Autodesk Inventor part; units mm, degrees
ref_plane "YZ Plane" through (0, 0, 0) normal (1, 0, 0) x (0, 1, 0)
ref_plane "XZ Plane" through (0, 0, 0) normal (0, 1, 0) x (-1, 0, 0)
ref_plane "XY Plane" through (0, 0, 0) normal (0, 0, 1) x (1, 0, 0)
sketch "Sketch1" plane through (0, 0, 0) normal (0, 1, 0) x (-1, 0, 0)
  line L0 (0, 0) -> (0, -90)
  line L1 (0, -90) -> (-5, -90)
  line L2 (-5, -90) -> (-5, -87.5)
  line L3 (-5, -82.5) -> (-5, -7.5)
  line L4 (-5, -7.5) -> (-7.5, -9)
  line L5 (-7.5, -9) -> (-7.5, -1)
  line L6 (-7.5, -1) -> (-5, -2.5)
  line L7 (-5, -2.5) -> (-5, 0)
  line L8 (-5, 0) -> (0, 0)
  line L9 (-5, -7.5) -> (-5, -2.5) construction
  line L10 (-5, -82.5) -> (-5, -87.5) construction
  line L11 (0, -45) -> (-5, -45) construction
  line L12 (-5, -82.5) -> (-7.5, -81)
  line L13 (-7.5, -81) -> (-7.5, -89)
  line L14 (-7.5, -89) -> (-5, -87.5)
  line L15 (0, 0) -> (-10, 0)
  line L16 (-10, 0) -> (-10, -10)
  line L17 (-10, -10) -> (0, -10)
  line L18 (0, -10) -> (0, 0)
  line L19 (0, -90) -> (-10, -90)
  line L20 (-10, -90) -> (-10, -80)
  line L21 (-10, -80) -> (0, -80)
  line L22 (0, -80) -> (0, -90)
  point P0 (-7.5, -5)
  point P1 (-5, -5)
  point P2 (-5, -85)
  point P3 (0, -80)
  point P4 (-5, 0)
  point P5 (0, -10)
  point P6 (-5, -80)
  dimension "d0" = 90
  dimension "d1" = 5
  dimension "d2" = 8
  dimension "d3" = 5
  dimension "d4" = 5
  dimension "d5" = 2.5
  dimension "d6" = 5
  dimension "d9" = 5
  dimension "d10" = 10
  dimension "d11" = 10
  dimension "d12" = 10
  dimension "d13" = 10
extrude "Extrusion1" add sketch "Sketch1" along normal blind 3 contours L0 L17 L3 L4 L5 L6 L7 L8 | L7 L6 L5 L4 L3 L17 L16 L15 | L0 L1 L2 L14 L13 L12 L3 L21 | L3 L12 L13 L14 L2 L19 L20 L21
extrude "Extrusion2" add sketch "Sketch1" along normal blind 80 contours L0 L17 L3 L4 L5 L6 L7 L8 | L0 L21 L3 L17 | L0 L1 L2 L14 L13 L12 L3 L21
sketch "Sketch2" plane through (0, 0, 0) normal (0, 0, 1) x (1, 0, 0)
  line L0 (0, 0) -> (0, 80)
  line L1 (0, 13.75) -> (2.5, 13.75)
  line L2 (2.5, 13.75) -> (2.5, 16.25)
  line L3 (2.5, 16.25) -> (0, 16.25)
  line L4 (0, 16.25) -> (0, 13.75)
  line L5 (0, 66.25) -> (2.5, 66.25)
  line L6 (2.5, 66.25) -> (2.5, 63.75)
  line L7 (2.5, 63.75) -> (0, 63.75)
  line L8 (0, 63.75) -> (0, 66.25)
  line L9 (0, 80) -> (5, 80)
  line L10 (0, 0) -> (10, 0)
  point P0 (2.5, 65)
  point P1 (2.5, 15)
  point P2 (0, 16.25)
  dimension "d18" = 15
  dimension "d19" = 2.5
  dimension "d20" = 2.5
  dimension "d21" = 15
  dimension "d22" = 2.5
extrude "Extrusion3" cut sketch "Sketch2" against normal up to surface (90 mm away)
sketch "Sketch3" plane through (0, 3, 0) normal (0, 1, 0) x (1, 0, 0)
  line L0 (5, 82.5) -> (5, 80)
  line L1 (5, 80) -> (10, 80)
  line L2 (10, 80) -> (10, 90)
  line L3 (10, 90) -> (5, 90)
  line L4 (5, 90) -> (5, 87.5)
  line L5 (5, 87.5) -> (7.5, 89)
  line L6 (7.5, 89) -> (7.5, 81)
  line L7 (7.5, 81) -> (5, 82.5)
  line L8 (5, 10) -> (5, 7.5)
  line L9 (5, 7.5) -> (7.5, 9)
  line L10 (7.5, 9) -> (7.5, 1)
  line L11 (7.5, 1) -> (5, 2.5)
  line L12 (5, 2.5) -> (5, 0)
  line L13 (5, 0) -> (10, 0)
  line L14 (10, 0) -> (10, 10)
  line L15 (10, 10) -> (5, 10)
  point P0 (0, 0)
extrude "Extrusion4" cut sketch "Sketch3" against normal blind 0.1
sketch "Sketch4" plane through (0, 80, 0) normal (0, 1, 0) x (1, 0, 0)
  line L0 (7.5, 89) -> (5, 87.5)
  line L1 (7.5, 81) -> (7.5, 89)
  line L2 (5, 82.5) -> (7.5, 81)
  line L3 (7.5, 9) -> (5, 7.5)
  line L4 (7.5, 1) -> (7.5, 9)
  line L5 (5, 2.5) -> (7.5, 1)
  line L6 (5, 7.3834) -> (7.4, 8.8234)
  line L7 (7.4, 8.8234) -> (7.4, 1.1766)
  line L8 (7.4, 1.1766) -> (5, 2.6166)
  line L9 (5, 82.6166) -> (7.4, 81.1766)
  line L10 (7.4, 81.1766) -> (7.4, 88.8234)
  line L11 (7.4, 88.8234) -> (5, 87.3834)
  line L12 (5, 7.5) -> (5, 82.5)
  line L13 (5, 87.5) -> (5, 82.5)
  line L14 (5, 7.5) -> (5, 2.5)
  point P0 (0, 0)
  dimension "d27" = 0.1
  dimension "d28" = 0.1
  dimension "d29" = 0.1
  dimension "d30" = 0.1
  dimension "d33" = 0.1
  dimension "d34" = 0.1
extrude "Extrusion5" cut sketch "Sketch4" against normal up to surface (77.1 mm away) contours L1 L2 L13 L9 L10 L11 L0 | L3 L4 L5 L14 L8 L7 L6
sketch "Sketch5" plane through (10, 0, -80) normal (1, 0, 0) x (0, 0, -1)
  line L0 (-70, 2.9) -> (-80, 2.9)
  line L1 (-80, 0) -> (-80, 2.9)
  line L2 (-80, 0) -> (-70, 0)
  line L3 (-70, 0) -> (-70, 2.9)
  line L4 (10, 2.9) -> (0, 2.9)
  line L5 (0, 0) -> (0, 2.9)
  line L6 (0, 0) -> (10, 0)
  line L7 (10, 0) -> (10, 2.9)
extrude "Extrusion6" cut sketch "Sketch5" against normal blind 0.1
sketch "Sketch6" plane through (9.9, 0, -80) normal (1, 0, 0) x (0, 0, -1)
  line L0 (10, 0) -> (-80, 0)
  line L1 (-71.1766, 2.9) -> (-78.8234, 2.9)
  line L2 (0.1, 0) -> (-70.1, 0)
  line L3 (-70.1, 0) -> (-70.1, 2.9)
  line L4 (-70.1, 2.9) -> (0.1, 2.9)
  line L5 (0.1, 2.9) -> (0.1, 0)
  line L6 (-70, 2.9) -> (-70, 0) construction
  line L7 (0, 0) -> (0, 2.9) construction
  point P0 (-70.1, 0)
  dimension "tol" = 0.1
  dimension "d38" = 0.1
extrude "Extrusion7" cut sketch "Sketch6" against normal up to surface (4.9 mm away)
sketch "Sketch7" plane through (0, 80, 0) normal (0, 1, 0) x (1, 0, 0)
  line L0 (5, 87.3834) -> (5, 90)
  line L1 (5, 90) -> (0, 90)
  line L2 (0, 90) -> (0, 0)
  line L3 (0, 0) -> (5, 0)
  line L4 (5, 0) -> (5, 2.6166)
  line L5 (5, 2.6166) -> (7.4, 1.1766)
  line L6 (7.4, 1.1766) -> (7.4, 8.8234)
  line L7 (7.4, 8.8234) -> (5, 7.3834)
  line L8 (5, 7.3834) -> (5, 82.6166)
  line L9 (5, 82.6166) -> (7.4, 81.1766)
  line L10 (7.4, 81.1766) -> (7.4, 88.8234)
  line L11 (7.4, 88.8234) -> (5, 87.3834)
extrude "Extrusion8" cut sketch "Sketch7" against normal blind 0.2
sketch "Sketch8" plane through (0, 0, 0) normal (0, -1, 0) x (1, 0, 0)
  line L0 (5, -9.9) -> (9.9, -9.9)
  line L1 (9.9, -9.9) -> (9.9, 0)
  line L2 (0, 0) -> (9.9, 0)
  line L3 (0, -90) -> (0, 0)
  line L4 (9.9, -90) -> (0, -90)
  line L5 (9.9, -90) -> (9.9, -80.1)
  line L6 (9.9, -80.1) -> (5, -80.1)
  line L7 (5, -80.1) -> (5, -9.9)
extrude "Extrusion9" cut sketch "Sketch8" against normal blind 0.2
sketch "Sketch9" plane through (0, 16.25, 0) normal (-1, 0, 0) x (0, 0, 1)
  line L0 (-90, 0) -> (0, 0)
  line L1 (0, 0) -> (0, 47.5)
  line L2 (0, 47.5) -> (-90, 47.5)
  line L3 (-90, 0) -> (-90, 47.5)
  line L4 (0, 63.55) -> (-90, 63.55)
  line L5 (-90, 50) -> (-90, 63.55)
  line L6 (-90, 50) -> (0, 50)
  line L7 (0, 50) -> (0, 63.55)
  line L8 (-90, -16.05) -> (0, -16.05)
  line L9 (0, -16.05) -> (0, -2.5)
  line L10 (0, -2.5) -> (-90, -2.5)
  line L11 (-90, -16.05) -> (-90, -2.5)
  point P0 (0, -16.25)
extrude "Extrusion10" cut sketch "Sketch9" against normal blind 0.2
equation "\"d25\" = tol"
equation "\"d27\" = tol"
equation "\"d28\" = tol"
equation "\"d29\" = tol"
equation "\"d30\" = tol"
equation "\"d33\" = tol"
equation "\"d34\" = tol"
equation "\"d35\" = tol"
equation "\"d38\" = tol"
equation "\"d41\" = 2 * tol"
equation "\"d43\" = 2 * tol"
equation "\"d45\" = 2 * tol"
properties part number "drawerside"
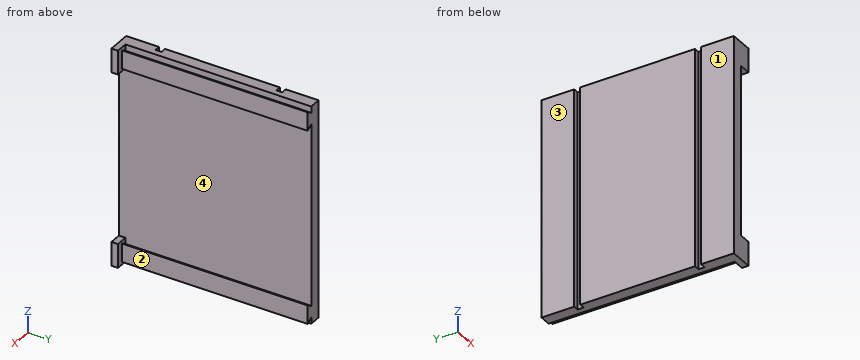
Check sheet for the modelled part. Datum: model origin and axes. Units: mm. Face numbers are marked on the shaded views. A direction names the side the tool comes from. Give positions to 0.01 mm unless a question says otherwise; leave off trailing zeros. Order: outer loops, then holes, each group sorted by start corner. A loop starts at its lowest first (then second) coordinate and runs counter-clockwise, first axis right, second up. Notation, with made-up numbers: M 44.5,-1 L 80.5,-1 A17 ccw 80.5,6 Z; hole C -11,32.5 d2. An arc over 180 degrees is marked long. Answer in a Markdown table with one row per item. Add a question column.
Q1. Release check for a two-part mould opening along Z. For the marked faces 3 and 4 record: released by +Z, released by -Z, zero draft, split by the parting line, or undercut.
Q2. Access from +Z, -Z, +X, -X, +Y, -Y to the whole of each face (thin tool, end or side, straight path). Record for the marked faces 1 and 2.
Q3. Sectioned sample at B-B, the plane y = 47.5. Record the boundary of the cut face in (x, z).
Q4. Thickness scan on L1, parallel to Y at x = 2.25, z = -24; L2, parallel to X at y = 18, z = -37; L3, parallel to Z at x = 5.75, y = 74.5. Record the ranges inside material, lowest first.
Q5. Gauge pin test, flat ends, axial feed: pin 1 Ø22.5 at (y, z) = (44.5, -37) entering from +X; pin 2 Ø1.3 at (y, z) = (36.5, -1.5) entering from +X. Record the tip position at first contact, or that the pin passes through.
Q6. Sectioned sample at A-A, the plane z = -15. Record the boundary of the cut face in (x, y).
Q7. Sectioned sample at C-C, the plane x = 6. Record the boundary of the cut face in (y, z).
Verdict:
| question | item | result |
|---|---|---|
| 1 | face 3 | zero draft |
| 1 | face 4 | undercut |
| 2 | face 1 | +Z, -Z, -X, +Y, -Y |
| 2 | face 2 | +Z, -Z, +X, +Y |
| 3 | outline | M 0.2,-90 L 5,-90 L 5,-87.38 L 7.4,-88.82 L 7.4,-81.18 L 5,-82.62 L 5,-7.38 L 7.4,-8.82 L 7.4,-1.18 L 5,-2.62 L 5,0 L 0.2,0 Z |
| 4 | L1 | 0.2 to 13.75, 16.25 to 63.75, 66.25 to 79.8 |
| 4 | L2 | 0.2 to 5 |
| 4 | L3 | -87.83 to -82.17, -7.83 to -2.17 |
| 5 | pin 1 | x = 5 |
| 5 | pin 2 | x = 7.4 |
| 6 | outline | M 0.2,0.2 L 5,0.2 L 5,79.8 L 0.2,79.8 L 0.2,66.25 L 2.5,66.25 L 2.5,63.75 L 0.2,63.75 L 0.2,16.25 L 2.5,16.25 L 2.5,13.75 L 0.2,13.75 Z |
| 7 | outline | M 0.2,-90 L 2.9,-90 L 2.9,-87.98 L 79.8,-87.98 L 79.8,-82.02 L 2.9,-82.02 L 2.9,-80.1 L 0.2,-80.1 Z; M 0.2,-9.9 L 2.9,-9.9 L 2.9,-7.98 L 79.8,-7.98 L 79.8,-2.02 L 2.9,-2.02 L 2.9,0 L 0.2,0 Z |
